```python
from build123d import *

# Parameters (mm, degrees)
PAD_DEPTH   = 2.5
FILLET_R    = 0.99
FILLET001_R = 0.99
FILLET002_R = 1.4
FILLET003_R = 2
FILLET004_R = 1
FILLET005_R = 2


with BuildPart() as part:
    # Sketch → Pad (new body)
    with BuildSketch(Plane.XY):
        Polygon((0, 0), (15, 10.503113), (16.720729, 8.045657), (-3, -5.762946), (-3, 3), (-9, 3), (-9, 6), (-3, 6), (-3, 27.5), (-12, 29.086943), (-12, 36.604242), (-9, 36.604242), (-9, 31.604242), (0, 30.017299), align=None)
    extrude(amount=PAD_DEPTH)

    # Fillet
    fillet_edges = [part.edges().sort_by_distance(p)[0] for p in [
        (-9, 3, 1.25),
        (-9, 6, 1.25),
    ]]
    fillet(fillet_edges, radius=FILLET_R)

    # Fillet001
    fillet001_edges = [part.edges().sort_by_distance(p)[0] for p in [
        (-12, 36.604242, 1.25),
        (-9, 36.604242, 1.25),
    ]]
    fillet(fillet001_edges, radius=FILLET001_R)

    # Fillet002
    fillet002_edges = [part.edges().sort_by_distance(p)[0] for p in [
        (15, 10.503113, 1.25),
        (16.720729, 8.045657, 1.25),
    ]]
    fillet(fillet002_edges, radius=FILLET002_R)

    # Fillet003
    fillet003_edges = [part.edges().sort_by_distance(p)[0] for p in [
        (0, 0, 1.25),
    ]]
    fillet(fillet003_edges, radius=FILLET003_R)

    # Fillet004
    fillet004_edges = [part.edges().sort_by_distance(p)[0] for p in [
        (-3, -5.762946, 1.25),
    ]]
    fillet(fillet004_edges, radius=FILLET004_R)

    # Fillet005
    fillet005_edges = [part.edges().sort_by_distance(p)[0] for p in [
        (-12, 29.086943, 1.25),
        (-3, 27.5, 1.25),
        (0, 30.017299, 1.25),
        (-9, 31.604242, 1.25),
    ]]
    fillet(fillet005_edges, radius=FILLET005_R)


solid = part.part
```
Geometry check sheet. Reference: the model listing, model coordinates, mm. A direction names the side the tool comes from. Round coordinates to 2 decimals unless told otherwise and drop trailing zeros. Order: outer loops, then holes, each group sorted by start corner. A loop starts at its lowest first (then second) coordinate and runs counter-clockwise, first axis right, second up. Notation, with made-up numbers: (-21, 83.5) - (-3, 83.5) arc R3 cw to (-3, 87.5) - close; hole circle Ø1 at (75, -39). An arc over 180 degrees is marked (long way). Use a Markdown table: item, result. Add a question column.
1) Set-up check for faces 4 (the flat face through (-9, 4.5, 1.2)), 5 (the cylindrical face through (-8.72, 5.7, 1.27)), 6 (the flat face through (7.19, 1.37, 1.23)), 7 (the cylindrical face through (-2.448, -4.736, 1.268)), 8 (the flat face through (-9, 34, 1)): record each of +Z, -Z, +X, -X, +Y, -Y from which the full face is reachable in a straight line by a thin tool's end or side.
2) Section check B-B (z = 1.5). Record the cut outline in (x, y), then the cut area to 4 significant figures.
3) Section check A-A (x = -6.5). Record the cut outline in (y, z).
4) Section check D-D (x = 4.5). Record the cut outline in (y, z).
5) Thickness scan on line 1 along X through (y, z) = (18, 1.75); line 2 along Y through (x, z) = (14.25, 0.5); line 3 along X through (y, z) = (5, 1). Record the ranges inside material, lowest first.
6) Mould release check, pull along Y, two halves, no side actions. Record for faces 1 (the cylindrical face through (16.15, 8.16, 1.27)), 2 (the flat face through (-7.46, 28.286, 1.232)), 3 (the flat face through (0, 16, 1)): released by +Y, released by -Y, zero draft, split by the parting line, or undercut.
7) Gauge pin test, flat ends, axial feed: P1, Ø0.8, axis at y = 0, z = 1, coming from the -X side; P2, Ø1, axis at x = 7, z = 1.5, coming from the +Y side. Record the tip position at first contact, or that the pin passes through.
8) Section check C-C (y = 16). Record the cut outline in (x, z), then the cut area to 3 significant figures.
Established:
| question | item | result |
|---|---|---|
| 1 | face 4 | +Z, -Z, -X, -Y |
| 1 | face 5 | +Z, -Z, -X |
| 1 | face 6 | +Z, -Z, +X, -Y |
| 1 | face 7 | +Z, -Z, -Y |
| 1 | face 8 | +Z, -Z, +X, +Y |
| 2 | outline | (-12, 30.77) arc R2 ccw to (-10.35, 28.8) - (-4.65, 27.79) arc R2 cw to (-3, 25.82) - (-3, 6) - (-8.01, 6) arc R0.99 ccw to (-9, 5.01) - (-9, 3.99) arc R0.99 ccw to (-8.01, 3) - (-3, 3) - (-3, -3.84) arc R1 ccw to (-1.43, -4.66) - (15.57, 7.24) arc R1.4 ccw to (15.92, 9.19) - (15.8, 9.36) arc R1.4 ccw to (13.85, 9.7) - (3.15, 2.2) arc R2 cw to (0, 3.84) - (0, 28.34) arc R2 ccw to (-1.65, 30.31) - (-7.35, 31.31) arc R2 cw to (-9, 33.28) - (-9, 35.61) arc R0.99 ccw to (-9.99, 36.6) - (-11.01, 36.6) arc R0.99 ccw to (-12, 35.61) - close |
| 2 | area | 223.5 mm2 |
| 3 | outline | (3, 0) - (6, 0) - (6, 2.5) - (3, 2.5) - close; (28.12, 0) - (31.16, 0) - (31.16, 2.5) - (28.12, 2.5) - close |
| 4 | outline | (-0.51, 0) - (3.15, 0) - (3.15, 2.5) - (-0.51, 2.5) - close |
| 5 | line 1 | -3 to 0 |
| 5 | line 2 | 6.32 to 9.89 |
| 5 | line 3 | -9 to 0, 7.14 to 12.37 |
| 6 | face 1 | split by the parting line |
| 6 | face 2 | undercut |
| 6 | face 3 | zero draft |
| 7 | P1 | x = -3 |
| 7 | P2 | y = 5.25 |
| 8 | outline | (-3, 0) - (0, 0) - (0, 2.5) - (-3, 2.5) - close |
| 8 | area | 7.50 mm2 |
